```python
from build123d import *

# Parameters (mm, degrees)
SKETCH2_W          = 1.9812
SKETCH2_H          = 6.35
CUT_EXTRUDE1_DEPTH = 1.27
FILLET1_R          = 0.3175


with BuildPart() as part:
    # Sketch2 → Revolve2 (revolve)
    with BuildSketch(Plane(origin=(0, 0, 0), x_dir=(0, 0, -1), z_dir=(1, 0, 0))):
        with BuildLine():
            Line((0, 9.144), (0, 7.7978))
            Line((0, 7.7978), (3.4544, 7.7978))
            add(Edge.make_bspline(
                [(1.905, 9.144), (2.485859984, 9.013201575), (3.169812282, 8.481844182), (3.4544, 7.7978)],
                knots=[0, 0, 0, 0, 1, 1, 1, 1], degree=3))
            Line((1.905, 9.144), (0, 9.144))
        make_face()
        Polygon((0, 7.7978), (0, 6.35), (1.9812, 6.35), (5.4229, 6.35), (5.4229, 7.7978), (3.4544, 7.7978), align=None)
        with Locations((0.9906, 3.175)):
            Rectangle(SKETCH2_W, SKETCH2_H)
        Polygon((1.9812, -5.152618014), (0, -6.35), (0, 0), (1.9812, 0), align=None)
    revolve(axis=Axis((0, 0, 0), (0, 1, 0)))

    # Sketch4 → Cut-Extrude1 (cut)
    with BuildSketch(Plane(origin=(0, 9.144, 0), x_dir=(1, 0, 0), z_dir=(0, 1, 0))):
        Polygon((-0.508, 2.228840954), (0.508, 2.228840954), (0.508, 0.884564976), (0.861964761, 0.530600214), (2.223569071, 0.530600214), (2.223569071, -0.530600214), (0.861964761, -0.530600214), (0.508, -0.884564976), (0.508, -2.228840954), (-0.508, -2.228840954), (-0.508, -0.884564976), (-0.861964761, -0.530600214), (-2.223569071, -0.530600214), (-2.223569071, 0.530600214), (-0.861964761, 0.530600214), (-0.508, 0.884564976), align=None)
    extrude(amount=-CUT_EXTRUDE1_DEPTH, mode=Mode.SUBTRACT)

    # Fillet1
    fillet1_edges = [part.edges().sort_by_distance(p)[0] for p in [
        (0, 7.7978, 5.4229),
    ]]
    fillet(fillet1_edges, radius=FILLET1_R)


solid = part.part
```
The listing builds one solid part. Answer for the finished solid, in the listing's coordinates (mm). A direction names the side the tool comes from. Give positions to 0.01 mm unless a question says otherwise; leave off trailing zeros. Order: outer loops, then holes, each group sorted by start corner. A loop starts at its lowest first (then second) coordinate and runs counter-clockwise, first axis right, second up. Notation, with made-up numbers: (25.5, 72.25) -> (52.5, 72.25) arc R8 ccw to (52.5, 80.25) -> close; hole circle Ø2 at (72, 66). An arc over 180 degrees is marked (long way). Answer as a JSON object with one key per item and string values. Group by question number.
Item 1: A tool of negligible diameter and unlimited length cuts with its end or side. For faces 1 (the cylindrical face through (5.294, 6.923, 1.176)), 2 (the flat face through (2.224, 8.5, 0)), 3 (the flat face through (-0.1, 6.35, 2.3)), from which of +Z, -Z, +X, -X, +Y, -Y can it reach the whole face along a straight path? Write none if from no direction.
Item 2: Flat-ended cylindrical pins translate along their axes: pin 1 (4 mm diameter, centred on x = -4, z = -1.5, fed in from +Y); pin 2 (1 mm diameter, centred on x = 1, y = 3, fed in from -Z); pin 3 (0.6 mm diameter, centred on x = -1.5, y = 8.5, fed in from +Z). Find the tip coordinate at first contact, or state that the pin passes through.
Item 3: The part is cut by section B-B on y = 4. Write down the section's boundary in (x, z).
Item 4: The part is cut by section A-A on y = 7. Write down the section's boundary in (x, z), and give its area (3 significant figures).
Item 5: Determine the mould class of faces 4 (the flat face through (0.508, 8.5, -1.6)), 5 (the cylindrical face through (-1.964, 0.679, 0.258)), 6 (the flat face through (-1, 9.144, -1)) for opening direction X: pulls with the +X half, pulls with the -X half, needs draft (parallel to the pull), parting line crosses it, or undercut.
Item 6: Consider L1, parallel to Y at x = -1.75, z = -4; L2, parallel to Z at x = 0, y = 2.5; L3, parallel to Z at x = -2, y = 8.5. Determine where each line is inside the solid, lowest interval first. Write a range as from..to.
Result set:
{
 "1": {"face 1": "+Y, -Y", "face 2": "+Y", "face 3": "-Y"},
 "2": {"pin 1": "y = 9.01", "pin 2": "z = -1.92", "pin 3": "z = 2.9"},
 "3": {"outline": "circle Ø3.96 at (0, 0)"},
 "4": {"outline": "circle Ø10.85 at (0, 0)", "area": "92.4 mm²"},
 "5": {"face 4": "undercut", "face 5": "parting line crosses it", "face 6": "needs draft"},
 "6": {"L1": "6.35..7.8", "L2": "-1.98..1.98", "L3": "-2.21..-0.53, 0.53..2.21"}
}
